Read the model definition and answer for the solid it produces. Units are mm, in the model's axes. Round coordinates to 2 decimals unless told otherwise and drop trailing zeros. Answer as a JSON object with one key per item and string values. Group by question number.
Q1. A cutting plane is placed at A-A on z = 1.25. Count the separate pieces of the cut face and the enclosed holes in it, and give its area (3 significant figures).
Q2. The mould has two halves that part along Y. Classify faces 1 (the cylindrical face through (-63.85, -99.75, 1.57)), 2 (the flat face through (14, 1, 3.175)): pulls with the +Y half, pulls with the -Y half, needs draft (parallel to the pull), parting line crosses it, or undercut.
Q3. Consider line 1 (X direction, y = -73.5, z = 1.15); line 2 (Y direction, x = 8, z = 0.2); line 3 (X direction, y = -26, z = 2.4). Determine where each line is inside the solid, lowest interval first.
Q4. Given pin 1 Ø2.5 at (x, y) = (-63.38, 73.77) entering from -Z, flat-ended and moving along its own axis, determine where the tip first touches the part or whether it passes through.
```python
from build123d import *

# Parameters (mm, degrees)
F0_W     = 134.69465
F0_H     = 206.984854
F0_R     = 2.15265
F0_R_2   = 1.25
F0_R_3   = 1.7272
F1_DEPTH = 3.175


with BuildPart() as f1:
    # F0 (on Top) → F1 (new body)
    with BuildSketch(Plane.XY):
        Rectangle(F0_W, F0_H)
        with Locations((-63.378575, -97.650427)):
            Circle(F0_R, mode=Mode.SUBTRACT)
        with Locations((-63.378575, -73.774427)):
            Circle(F0_R, mode=Mode.SUBTRACT)
        with Locations((-4.750003, -96.192416)):
            Circle(F0_R_2, mode=Mode.SUBTRACT)
        with Locations((-4.8895, -24.892)):
            Circle(F0_R_3, mode=Mode.SUBTRACT)
        with Locations((4.750003, -96.192416)):
            Circle(F0_R_2, mode=Mode.SUBTRACT)
        with Locations((63.378575, -97.650427)):
            Circle(F0_R, mode=Mode.SUBTRACT)
        with Locations((63.378575, -73.774427)):
            Circle(F0_R, mode=Mode.SUBTRACT)
        with Locations((4.8895, -24.892)):
            Circle(F0_R_3, mode=Mode.SUBTRACT)
        with BuildLine():
            Line((-1.016, -20.32), (-9.779, -20.32))
            Line((-9.779, -20.32), (-9.779, 20.32))
            Line((-9.779, 20.32), (-1.016, 20.32))
            Line((-1.016, 20.32), (-1.016, 23.749))
            ThreePointArc((-1.016, 23.749), (0, 24.765), (1.016, 23.749))
            Line((1.016, 23.749), (1.016, 20.32))
            Line((1.016, 20.32), (9.779, 20.32))
            Line((9.779, 20.32), (9.779, -20.32))
            Line((9.779, -20.32), (1.016, -20.32))
            Line((1.016, -20.32), (1.016, -23.749))
            ThreePointArc((1.016, -23.749), (0, -24.765), (-1.016, -23.749))
            Line((-1.016, -23.749), (-1.016, -20.32))
        make_face(mode=Mode.SUBTRACT)
        with Locations((-4.8895, 24.892)):
            Circle(F0_R_3, mode=Mode.SUBTRACT)
        with Locations((-63.378575, 73.774427)):
            Circle(F0_R, mode=Mode.SUBTRACT)
        with Locations((-63.378575, 97.650427)):
            Circle(F0_R, mode=Mode.SUBTRACT)
        with Locations((-4.750003, 96.192416)):
            Circle(F0_R_2, mode=Mode.SUBTRACT)
        with Locations((4.8895, 24.892)):
            Circle(F0_R_3, mode=Mode.SUBTRACT)
        with Locations((4.750003, 96.192416)):
            Circle(F0_R_2, mode=Mode.SUBTRACT)
        with Locations((63.378575, 73.774427)):
            Circle(F0_R, mode=Mode.SUBTRACT)
        with Locations((63.378575, 97.650427)):
            Circle(F0_R, mode=Mode.SUBTRACT)
    extrude(amount=F1_DEPTH)


solid = f1.part
```
Result set:
{
 "1": {"separate pieces": "1", "enclosed holes": "17", "area": "26,900 mm²"},
 "2": {"face 1": "undercut", "face 2": "needs draft"},
 "3": {"line 1": "x = -67.35 to -65.51, -61.24 to 61.24, 65.51 to 67.35", "line 2": "y = -103.49 to -20.32, 20.32 to 103.49", "line 3": "x = -67.35 to -6.21, -3.56 to 3.56, 6.21 to 67.35"},
 "4": {"pin 1": "passes through"}
}
